```python
from build123d import *

# Parameters (mm, degrees)
SKETCH1_W               = 20
SKETCH1_H               = 25
BOSS_EXTRUDE1_DEPTH     = 17
CUT_EXTRUDE1_DEPTH      = 32.843366656
BOSS_EXTRUDE2_DEPTH     = 5
SKETCH4_R               = 2
CUT_EXTRUDE2_DEPTH      = 37.249137921
SKETCH6_W               = 20
SKETCH6_H               = 20
BOSS_EXTRUDE3_DEPTH     = 7
SKETCH8_W               = 8.2
SKETCH8_H               = 3.8
CUT_EXTRUDE3_DEPTH      = 41.401113846
CUT_EXTRUDE4_REACH      = 43.379
CUT_EXTRUDE4_END_RADIUS = 7
SKETCH7_R               = 2
SKETCH9_W               = 15
SKETCH9_H               = 7.5
CUT_EXTRUDE5_DEPTH      = 2
SKETCH10_W              = 10
SKETCH10_H              = 0.75
CUT_EXTRUDE6_DEPTH      = 41.01249811


with BuildPart() as part:
    # Sketch1 → Boss-Extrude1 (new body)
    with BuildSketch(Plane(origin=(0, 0, 0), x_dir=(1, 0, 0), z_dir=(0, 1, 0))):
        Rectangle(SKETCH1_W, SKETCH1_H)
    extrude(amount=BOSS_EXTRUDE1_DEPTH)

    # Sketch2 → Cut-Extrude1 (cut, through all)
    with BuildSketch(Plane.XY.offset(12.5)):
        with BuildLine():
            Line((0, 2), (-6.062177826, 5.5))
            ThreePointArc((-6.062177826, 5.5), (0, 16), (6.062177826, 5.5))
            Line((6.062177826, 5.5), (0, 2))
        make_face()
    extrude(amount=-CUT_EXTRUDE1_DEPTH, mode=Mode.SUBTRACT)

    # Sketch3 → Boss-Extrude2 (add)
    with BuildSketch(Plane.XY.offset(12.5)):
        Polygon((10, 0), (20, 0), (20, -10), (-20, -10), (-20, 0), (-10, 0), align=None)
    boss_extrude2 = extrude(amount=-BOSS_EXTRUDE2_DEPTH)

    # Mirror1: Boss-Extrude2 across plane
    add(boss_extrude2.mirror(Plane.XY))

    # Sketch4 → Cut-Extrude2 (cut, through all)
    with BuildSketch(Plane.XY.offset(12.5)):
        with Locations((16, -5)):
            Circle(SKETCH4_R)
        with Locations((-16, -5)):
            Circle(SKETCH4_R)
    extrude(amount=-CUT_EXTRUDE2_DEPTH, mode=Mode.SUBTRACT)

    # Sketch6 → Boss-Extrude3 (add)
    with BuildSketch(Plane(origin=(0, 17, 0), x_dir=(1, 0, 0), z_dir=(0, 1, 0))):
        Rectangle(SKETCH6_W, SKETCH6_H)
    extrude(amount=BOSS_EXTRUDE3_DEPTH)

    # Sketch8 → Cut-Extrude3 (cut, through all)
    with BuildSketch(Plane(origin=(10, 0, 0), x_dir=(0, 0, -1), z_dir=(1, 0, 0))):
        with Locations((0, 18.9)):
            Rectangle(SKETCH8_W, SKETCH8_H)
    extrude(amount=-CUT_EXTRUDE3_DEPTH, mode=Mode.SUBTRACT)

    # Cut-Extrude4: up to this cylinder (the profile starts outside it)
    cut_extrude4_end = Plane(origin=(0, 9, 0), z_dir=(0, 0, 1)) * Cylinder(CUT_EXTRUDE4_END_RADIUS, 101.758, mode=Mode.PRIVATE)
    # Sketch7 → Cut-Extrude4 (cut, up to the surface)
    with BuildSketch(Plane(origin=(0, 24, 0), x_dir=(1, 0, 0), z_dir=(0, 1, 0)), mode=Mode.PRIVATE) as cut_extrude4_sk1:
        with Locations(Location((0, 0, 0), (0, 0, 270))):
            Circle(SKETCH7_R)
    cut_extrude4_tool1 = extrude(cut_extrude4_sk1.sketch, amount=-CUT_EXTRUDE4_REACH, mode=Mode.PRIVATE) - cut_extrude4_end
    add(cut_extrude4_tool1.solids().sort_by_distance((0, 24, 0))[0], mode=Mode.SUBTRACT)

    # Sketch9 → Cut-Extrude5 (cut)
    with BuildSketch(Plane.ZY.offset(-10)):
        with Locations((0, 3.75)):
            Rectangle(SKETCH9_W, SKETCH9_H)
    extrude(amount=CUT_EXTRUDE5_DEPTH, mode=Mode.SUBTRACT)

    # Sketch10 → Cut-Extrude6 (cut, through all)
    with BuildSketch(Plane.XY.offset(12.5)):
        with Locations((-15, -5)):
            Rectangle(SKETCH10_W, SKETCH10_H)
        with Locations((15, -5)):
            Rectangle(SKETCH10_W, SKETCH10_H)
    extrude(amount=-CUT_EXTRUDE6_DEPTH, mode=Mode.SUBTRACT)


solid = part.part
```
For this review, take the finished solid that the model builds, in its own axes (mm). A direction names the side the tool comes from. Round coordinates to 2 decimals unless told otherwise and drop trailing zeros. Write each loop counter-clockwise with the first axis right and the second up, starting at its lowest first coordinate (ties: lowest second). Pieces come first, ordered by that corner, then holes. Notation, with made-up numbers: (84.5, 55) -> (143.5, 55) arc R9 cw to (143.5, 64) -> close; hole circle Ø5 at (52.25, -20.5). An arc over 180 degrees is marked (long way). Use one line per item in the form item = value.
1) Take a section at D-D, the plane x = -13.5. Write out the cut boundary in (y, z) (3 decimals).
Found:
outline = (-10, -12.5) -> (-5.375, -12.5) -> (-5.375, -7.5) -> (-10, -7.5) -> close; (-10, 7.5) -> (-5.375, 7.5) -> (-5.375, 12.5) -> (-10, 12.5) -> close; (-4.625, -12.5) -> (0, -12.5) -> (0, -7.5) -> (-4.625, -7.5) -> close; (-4.625, 7.5) -> (0, 7.5) -> (0, 12.5) -> (-4.625, 12.5) -> close
2) Clearance check with flat-ended pins moving along their axes: pin 1 (10 mm diameter, centred on y = 9, z = 1, fed in from +X); pin 2 (2 mm diameter, centred on y = 18.5, z = -0.5, fed in from -X); pin 3 (0.6 mm diameter, centred on x = 19, z = -11, fed in from +Y); pin 4 (6 mm diameter, centred on x = 11.5, z = 3, fed in from -Y). State where each tip first meets the part, or that it passes through.
Found:
pin_1 = 10
pin_2 = through
pin_3 = 0
pin_4 = 7.5
3) Take a section at B-B, the plane y = 9. Write out the cut boundary in (x, z).
Found:
outline = (-10, -12.5) -> (-7, -12.5) -> (-7, 12.5) -> (-10, 12.5) -> close; (7, -12.5) -> (10, -12.5) -> (10, 12.5) -> (7, 12.5) -> close
4) Take a section at A-A, the plane z = 3.25. Write out the cut boundary in (x, y), and give its area (3 significant figures).
Found:
outline = (-10, 0) -> (8, 0) -> (8, 7.5) -> (10, 7.5) -> (10, 17) -> (-10, 17) -> close; (-10, 20.8) -> (10, 20.8) -> (10, 24) -> (-10, 24) -> close; hole (-6.06, 5.5) -> (0, 2) -> (6.06, 5.5) arc R7 ccw (long way) to start
area = 244 mm2
5) Tool access review of faces 4 (the cylindrical face through (-1.2, 16.4, -1.6)), 5 (the flat face through (0, 19, -4.1)), 6 (the flat face through (-19, -4.625, 10)), 7 (the cylindrical face through (16, -3, -10)), 8 (the flat face through (15, 0, -10)): name each direction out of +Z, -Z, +X, -X, +Y, -Y from which nothing blocks a thin tool from reaching the whole face with its end or side.
Found:
face_4 = +Y
face_5 = +X, -X
face_6 = +Z, -Z, -X
face_7 = +Z, -Z
face_8 = +Z, -Z, +X, +Y
6) Take a section at C-C, the plane z = 0. Write out the cut boundary in (x, y).
Found:
outline = (-10, 0) -> (8, 0) -> (8, 7.5) -> (10, 7.5) -> (10, 17) -> (2, 17) -> (2, 15.71) arc R7 cw to (6.06, 5.5) -> (0, 2) -> (-6.06, 5.5) arc R7 cw to (-2, 15.71) -> (-2, 17) -> (-10, 17) -> close; (-10, 20.8) -> (-2, 20.8) -> (-2, 24) -> (-10, 24) -> close; (2, 20.8) -> (10, 20.8) -> (10, 24) -> (2, 24) -> close
7) Mouldability with a two-part tool opening along Y and no side actions: class faces 1 (the flat face through (-15, 0, 10)), 2 (the flat face through (20, -2, -10)), 3 (the cylindrical face through (16, -7, -10)) as +Y half, -Y half, draft (parallel to the pull), parting line (faces both ways), or undercut.
Found:
face_1 = +Y half
face_2 = draft
face_3 = undercut
8) To check wall thickness, follow L1, parallel to Z at x = 0, y = 16.75; L2, parallel to Z at x = -12, y = -3.5; L3, parallel to X at y = 9, z = -7.25. State the ranges of each line that lie inside material, in increasing order. Write a range as from..to.
Found:
L1 = -12.5..-2, 2..12.5
L2 = -12.5..-7.5, 7.5..12.5
L3 = -10..-7, 7..10
